Geometry check sheet. Reference: drawing and pictorial views, mm from the part's lowest x, y, z. Coordinates: 2 decimals unless noted, no trailing zeros. Loops run counter-clockwise (first coordinate to the right, second up) from the corner with the lowest first, then second, coordinate; pieces in that order, holes last. Notation, with made-up numbers: (-37, -12) -> (-33, -12) arc R26 cw to (-33, 3) -> close; hole circle Ø9 at (-2, 53.25). An arc over 180 degrees is marked (long way). Answer as a JSON object with one key per item and string values. Group by question number.
Q1. Scan lines: L1, parallel to Z at x = 609.6, y = 21; L2, parallel to X at y = 12, z = 609; L3, parallel to Z at x = 660, y = 8. Record each from-to range of solid material in increasing order.
Q2. Cross-section at A-A on y = 28. Record the boundary of the cut face in (x, z), and give its area (3 significant figures).
Q3. Cross-section at C-C on x = 213. Record the boundary of the cut face in (y, z).
Q4. Gauge pin test, flat ends, axial feed: pin 1 Ø3 at (x, y) = (316.5, 33.5) entering from -Z; pin 2 Ø1.5 at (x, y) = (262, 33) entering from +Z; pin 3 Ø10 at (y, z) = (17, 1045.5) entering from -X; pin 4 Ø12 at (x, z) = (406, 853) entering from -Y. Record the tip position at first contact, or that the pin passes through.
Q5. Cross-section at B-B on z = 247.5. Record the boundary of the cut face in (x, y).
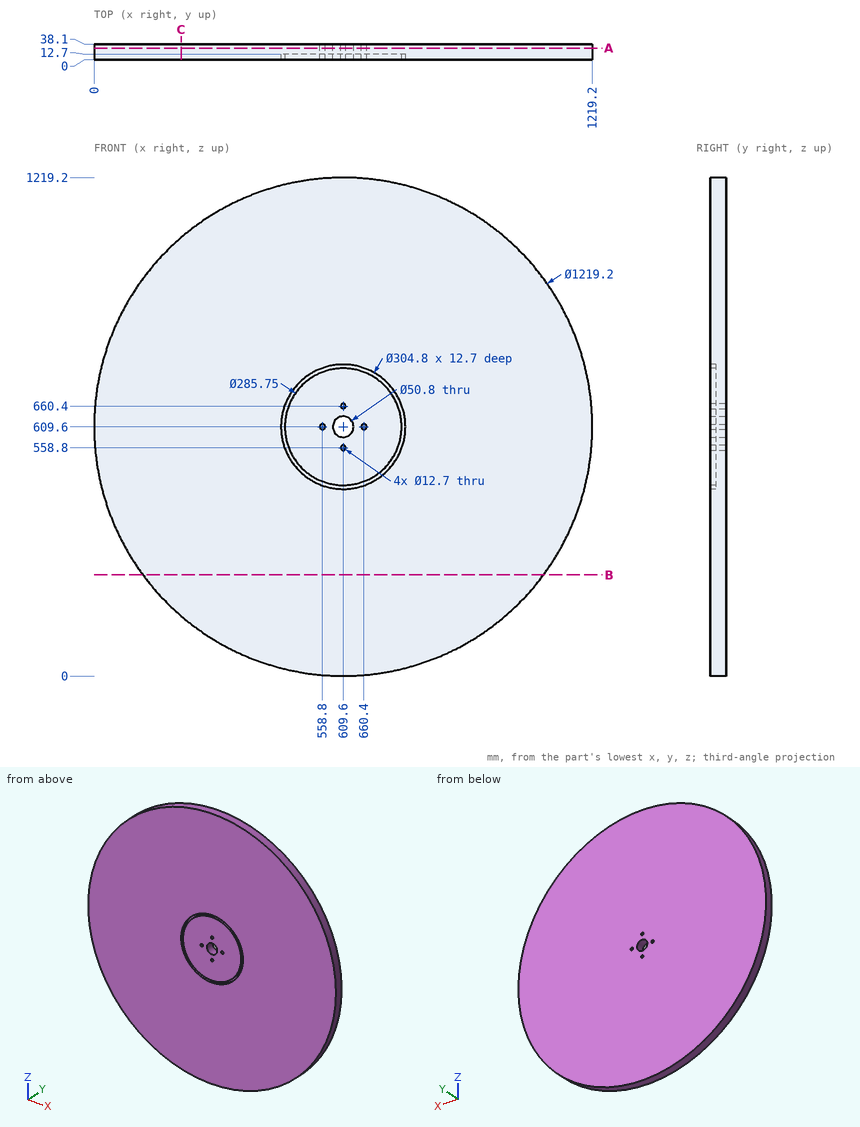
Computed values:
{
 "1": {"L1": "z = 0 to 552.45, 565.15 to 584.2, 635 to 654.05, 666.75 to 1219.2", "L2": "x = 0 to 457.2, 466.73 to 552.48, 565.12 to 584.21, 634.99 to 654.08, 666.72 to 752.47, 762 to 1219.2", "L3": "z = 2.09 to 465.78, 475.91 to 603.26, 615.94 to 743.29, 753.42 to 1217.11"},
 "2": {"outline": "circle Ø1219.2 at (609.6, 609.6); hole circle Ø12.7 at (558.8, 609.6); hole circle Ø50.8 at (609.6, 609.6); hole circle Ø12.7 at (609.6, 558.8); hole circle Ø12.7 at (609.6, 660.4); hole circle Ø12.7 at (660.4, 609.6)", "area": "1,160,000 mm²"},
 "3": {"outline": "(0, 146.65) -> (38.1, 146.65) -> (38.1, 1072.55) -> (0, 1072.55) -> close"},
 "4": {"pin 1": "stops at z = 74.27", "pin 2": "stops at z = 1110.91", "pin 3": "stops at x = 178.4", "pin 4": "stops at y = 0"},
 "5": {"outline": "(119.2, 0) -> (1100, 0) -> (1100, 38.1) -> (119.2, 38.1) -> close"}
}
